Input: part model. Units: mm. Frame: model coordinates. Give positions to 0.01 mm unless a question says otherwise; leave off trailing zeros. Write each loop counter-clockwise with the first axis right and the second up, starting at its lowest first coordinate (ties: lowest second). Pieces come first, ordered by that corner, then holes.
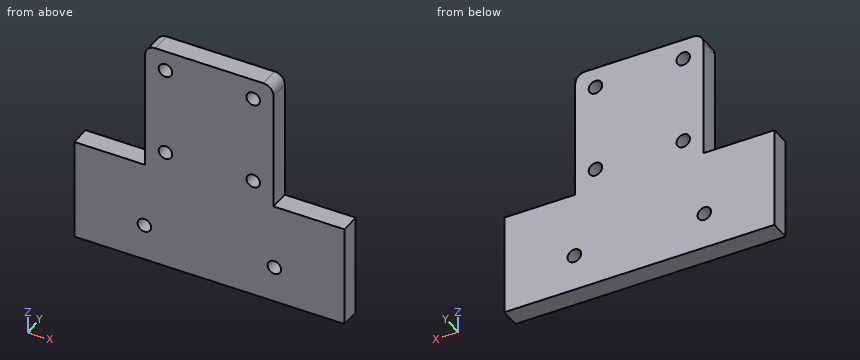
```python
from build123d import *

# Parameters (mm, degrees)
SKETCH1_W            = 38
SKETCH1_H            = 38
BOSS_EXTRUDE1_DEPTH  = 6
SKETCH2_R            = 2
CUT_EXTRUDE1_DEPTH   = 55.074023338
LPATTERN1_COUNT      = 2
LPATTERN1_PITCH      = 26
LPATTERN1_COUNT_DIR2 = 2
LPATTERN1_PITCH_DIR2 = 26
FILLET1_R            = 3
BOSS_EXTRUDE2_DEPTH  = 6
SKETCH4_R            = 2
CUT_EXTRUDE2_DEPTH   = 91.227490268


with BuildPart() as part:
    # Sketch1 → Boss-Extrude1 (new body)
    with BuildSketch(Plane(origin=(0, 0, 0), x_dir=(1, 0, 0), z_dir=(0, 1, 0))):
        with Locations((19, 19)):
            Rectangle(SKETCH1_W, SKETCH1_H)
    extrude(amount=BOSS_EXTRUDE1_DEPTH)

    # Sketch2 → Cut-Extrude1 (cut, through all)
    with BuildSketch(Plane(origin=(0, 6, 0), x_dir=(1, 0, 0), z_dir=(0, 1, 0))):
        with Locations(Location((6, 32, 0), (0, 0, 270))):
            Circle(SKETCH2_R)
    cut_extrude1 = extrude(amount=-CUT_EXTRUDE1_DEPTH, mode=Mode.SUBTRACT)

    # LPattern1: Cut-Extrude1 2 × 2
    with Locations(*[(i * LPATTERN1_PITCH, 0, j * LPATTERN1_PITCH_DIR2) for i in range(LPATTERN1_COUNT) for j in range(LPATTERN1_COUNT_DIR2) if (i, j) != (0, 0)]):
        add(cut_extrude1, mode=Mode.SUBTRACT)

    # Fillet1
    fillet1_edges = [part.edges().sort_by_distance(p)[0] for p in [
        (38, 3, 0),
        (0, 3, 0),
    ]]
    fillet(fillet1_edges, radius=FILLET1_R)

    # Sketch3 → Boss-Extrude2 (add)
    with BuildSketch(Plane(origin=(0, 0, 0), x_dir=(1, 0, 0), z_dir=(0, 1, 0))):
        Polygon((0, 38), (-21, 38), (-21, 68), (59, 68), (59, 38), (38, 38), align=None)
    extrude(amount=BOSS_EXTRUDE2_DEPTH)

    # Sketch4 → Cut-Extrude2 (cut, through all)
    with BuildSketch(Plane(origin=(0, 6, 0), x_dir=(1, 0, 0), z_dir=(0, 1, 0))):
        with Locations(Location((-0.25, 57.25, 0), (0, 0, 270))):
            Circle(SKETCH4_R)
        with Locations(Location((38.25, 57.25, 0), (0, 0, 270))):
            Circle(SKETCH4_R)
    extrude(amount=-CUT_EXTRUDE2_DEPTH, mode=Mode.SUBTRACT)


solid = part.part
```
Q1. Pin query (flat end, axial travel): pin 1 (1 mm diameter, centred on y = 3, z = -32.5, fed in from +X); pin 2 (1.5 mm diameter, centred on x = 41.5, y = 2.5, fed in from +Z). Return the tip coordinate at first contact, or that it passes through.
Q2. Material intervals for line 1 along X through (y, z) = (3, -6); line 2 along X through (y, z) = (1.9, -57.25); line 3 along X through (y, z) = (3.6, -18.5), sorted ascending.
Q3. Section C-C, the plane y = 4.7. Return the cut outline in (x, z), then the cut area to 3 significant figures.
Q4. Section B-B, the plane x = 32. Return the cut outline in (y, z), then the cut area to 3 significant figures.
Q5. Section A-A, the plane z = -57.25. Return the cut outline in (x, y), then the cut area to 3 significant figures.
Q6. Section D-D, the plane x = -12.5. Return the cut outline in (y, z).
Solutions:
1. pin 1: stops at x = 38
1. pin 2: stops at z = -38
2. line 1: x = 0 to 4, 8 to 30, 34 to 38
2. line 2: x = -21 to -2.25, 1.75 to 36.25, 40.25 to 59
2. line 3: x = 0 to 38
3. outline: (-21, -68) - (59, -68) - (59, -38) - (38, -38) - (38, -3) arc R3 ccw to (35, 0) - (3, 0) arc R3 ccw to (0, -3) - (0, -38) - (-21, -38) - close; hole circle Ø4 at (-0.25, -57.25); hole circle Ø4 at (6, -32); hole circle Ø4 at (6, -6); hole circle Ø4 at (32, -32); hole circle Ø4 at (32, -6); hole circle Ø4 at (38.25, -57.25)
3. area: 3,760 mm2
4. outline: (0, -68) - (6, -68) - (6, -34) - (0, -34) - close; (0, -30) - (6, -30) - (6, -8) - (0, -8) - close; (0, -4) - (6, -4) - (6, 0) - (0, 0) - close
4. area: 360 mm2
5. outline: (-21, 0) - (-2.25, 0) - (-2.25, 6) - (-21, 6) - close; (1.75, 0) - (36.25, 0) - (36.25, 6) - (1.75, 6) - close; (40.25, 0) - (59, 0) - (59, 6) - (40.25, 6) - close
5. area: 432 mm2
6. outline: (0, -68) - (6, -68) - (6, -38) - (0, -38) - close
